For this review, take the finished solid that the model builds, in its own axes (mm). A direction names the side the tool comes from. Coordinates: 2 decimals unless noted, no trailing zeros. Write each loop counter-clockwise with the first axis right and the second up, starting at its lowest first coordinate (ties: lowest second). Pieces come first, ordered by that corner, then holes. Notation, with made-up numbers: (-37, 2) - (19, 2) arc R12 ccw to (19, 22) - close; hole circle Ø3 at (63.5, 23). An arc over 180 degrees is marked (long way). Write each question's results on one line, items separated by ' | '.
from build123d import *

# Parameters (mm, degrees)
PAD_DEPTH        = 5
SKETCH004_R      = 3
POCKET_DEPTH     = 3
HOLE_D           = 2.4
HOLE_CSINK_D     = 4
HOLE_CSINK_ANGLE = 90
SKETCH006_W      = 5
SKETCH006_H      = 10
PAD001_DEPTH     = 20
SKETCH007_W      = 5
SKETCH007_H      = 10
PAD002_DEPTH     = 20
SKETCH008_R      = 1.2
HOLE001_DEPTH    = 66.882828


with BuildPart() as part:
    # Sketch → Pad (new body)
    with BuildSketch(Plane.XY):
        with BuildLine():
            ThreePointArc((-9.299092, 37.700908), (-7.543295, 36.530982), (-5.472396, 36.127344))
            Line((-5.472396, 36.127344), (5.472396, 36.127344))
            ThreePointArc((5.472396, 36.127344), (7.543295, 36.530982), (9.299092, 37.700908))
            Line((9.299092, 37.700908), (22.895203, 51.297019))
            Line((22.895203, 51.297019), (48.881828, 51.297019))
            Line((48.881828, 51.297019), (48.881828, 57.158768))
            Line((-48.578125, 57.158768), (48.881828, 57.158768))
            Line((-48.578125, 51.297019), (-48.578125, 57.158768))
            Line((-22.895203, 51.297019), (-48.578125, 51.297019))
            Line((-9.299092, 37.700908), (-22.895203, 51.297019))
        make_face()
    extrude(amount=PAD_DEPTH)

    # Sketch004 (on Face11 of Pad) → Pocket (cut)
    with BuildSketch(Plane(origin=(0, 0, 0), x_dir=(1, 0, 0), z_dir=(0, 0, -1))):
        with Locations((-5.5, -41.5)):
            Circle(SKETCH004_R)
        with Locations((5.5, -41.5)):
            Circle(SKETCH004_R)
    extrude(amount=-POCKET_DEPTH, mode=Mode.SUBTRACT)

    # Hole (through all)
    with Locations(Plane.XY.offset(5)):
        with Locations((-5.5, 41.5), (5.5, 41.5)):
            CounterSinkHole(HOLE_D / 2, HOLE_CSINK_D / 2, counter_sink_angle=HOLE_CSINK_ANGLE)

    # Sketch006 (on Face5 of Hole) → Pad001 (join)
    with BuildSketch(Plane.XY.offset(5)):
        with Locations((-15.5, 52.158768)):
            Rectangle(SKETCH006_W, SKETCH006_H)
    extrude(amount=PAD001_DEPTH)

    # Sketch007 (on Face5 of Pad001) → Pad002 (join)
    with BuildSketch(Plane.XY.offset(5)):
        with Locations((15.5, 52.158768)):
            Rectangle(SKETCH007_W, SKETCH007_H)
    extrude(amount=PAD002_DEPTH)

    # Sketch008 (on Face15 of Pad002) → Hole001 (cut, through all)
    with BuildSketch(Plane(origin=(-18, 0, 0), x_dir=(0, -1, 0), z_dir=(-1, 0, 0))):
        with Locations((-52.158768, 22)):
            Circle(SKETCH008_R)
    extrude(amount=-HOLE001_DEPTH, mode=Mode.SUBTRACT)


solid = part.part
Q1. For pin 1 (8 mm diameter, centred on y = 53.5, z = 19, fed in from +X); pin 2 (11 mm diameter, centred on y = 51.5, z = 18, fed in from -X); pin 3 (2 mm diameter, centred on x = -5.5, y = 41.5, fed in from -Z); pin 4 (3.5 mm diameter, centred on x = -5.5, y = 41.5, fed in from -Z), all flat-tipped, find the tip position at first contact; note any pin that passes through.
Results found:
pin 1: x = 18 | pin 2: x = -18 | pin 3: through | pin 4: z = 3
Q2. Take a section at C-C on y = 41.5. State the section outline as (x, z) points, plus the area to 3 significant figures.
Results found:
outline: (-13.1, 0) - (-8.5, 0) - (-8.5, 3) - (-6.7, 3) - (-6.7, 4.2) - (-7.5, 5) - (-13.1, 5) - close; (-4.3, 3) - (-2.5, 3) - (-2.5, 0) - (2.5, 0) - (2.5, 3) - (4.3, 3) - (4.3, 4.2) - (3.5, 5) - (-3.5, 5) - (-4.3, 4.2) - close; (6.7, 3) - (8.5, 3) - (8.5, 0) - (13.1, 0) - (13.1, 5) - (7.5, 5) - (6.7, 4.2) - close | area: 84.1 mm2
Q3. Take a section at B-B on z = 22. State the section outline as (x, y) points, plus the area to 3 significant figures.
Results found:
outline: (-18, 47.16) - (-13, 47.16) - (-13, 50.96) - (-18, 50.96) - close; (-18, 53.36) - (-13, 53.36) - (-13, 57.16) - (-18, 57.16) - close; (13, 47.16) - (18, 47.16) - (18, 50.96) - (13, 50.96) - close; (13, 53.36) - (18, 53.36) - (18, 57.16) - (13, 57.16) - close | area: 76.0 mm2
Q4. Take a section at D-D on y = 54.25. State the section outline as (x, z) points, plus the area to 3 significant figures.
Results found:
outline: (-48.58, 0) - (48.88, 0) - (48.88, 5) - (18, 5) - (18, 25) - (13, 25) - (13, 5) - (-13, 5) - (-13, 25) - (-18, 25) - (-18, 5) - (-48.58, 5) - close | area: 687 mm2
Q5. Take a section at A-A on z = 14. State the section outline as (x, y) points, plus the area to 3 significant figures.
Results found:
outline: (-18, 47.16) - (-13, 47.16) - (-13, 57.16) - (-18, 57.16) - close; (13, 47.16) - (18, 47.16) - (18, 57.16) - (13, 57.16) - close | area: 100 mm2
Q6. For faces 4 (the face through (-18, 52, 15)), 5 (the face through (-36, 51.297, 2)), 6 (the face through (-5.891, 38.526, 1.479)), 7 (the face through (36, 51.297, 2)), 8 (the face through (18, 52, 15)), list the 3-axis set-ups (+Z, -Z, +X, -X, +Y, -Y) from which the entire face can be reached by the end or side of a thin tool; tool diameter is ignored.
Results found:
face 4: +Z, -X, +Y, -Y | face 5: +Z, -Z, -X, -Y | face 6: -Z | face 7: +Z, -Z, +X, -Y | face 8: +Z, +X, +Y, -Y
Q7. Wall thickness on line 1 along X through (y, z) = (50.75, 14.25); line 2 along Y through (x, z) = (-5.5, 3.9); line 3 along X through (y, z) = (41.5, 2.3): over which ranges is each line inside the solid? List them lowest first. Write a range as from..to.
Results found:
line 1: -18..-13, 13..18 | line 2: 36.13..40.3, 42.7..57.16 | line 3: -13.1..-8.5, -2.5..2.5, 8.5..13.1
Q8. Mouldability with a two-part tool opening along Y and no side actions: class faces 1 (the face through (-1, 49, 0)), 2 (the face through (-15.54, 51.05, 21.54)), 3 (the face through (-16, 47.159, 15)) as pulls with the +Y half, pulls with the -Y half, needs draft (parallel to the pull), parting line crosses it, or undercut.
Results found:
face 1: needs draft | face 2: undercut | face 3: pulls with the -Y half
